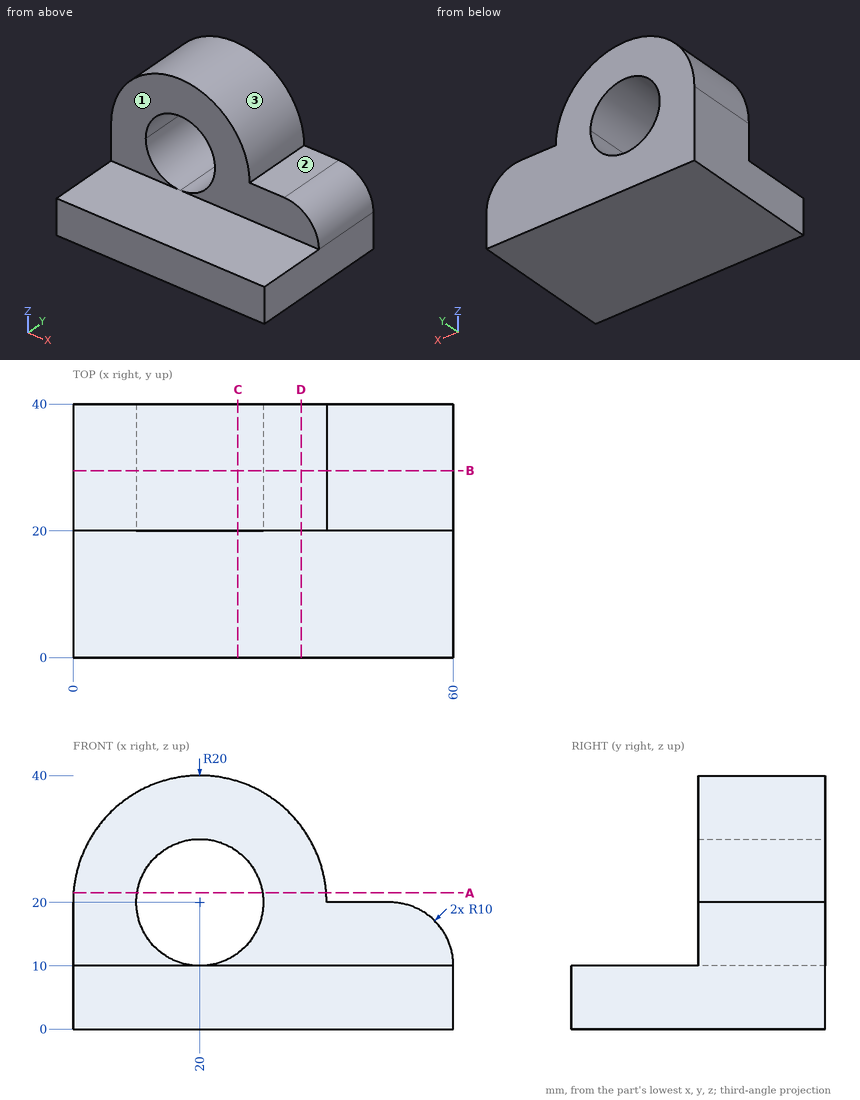
Geometry check sheet. Reference: drawing and pictorial views, mm from the part's lowest x, y, z. A direction names the side the tool comes from. Coordinates: 2 decimals unless noted, no trailing zeros. Order: outer loops, then holes, each group sorted by start corner. A loop starts at its lowest first (then second) coordinate and runs counter-clockwise, first axis right, second up.
Item 1: Section check A-A (z = 21.5). Enter the section's corners in (x, y), plus the area to 3 significant figures.
Item 2: Section check B-B (y = 29.5). Enter the section's corners in (x, z).
Item 3: Scan lines: line 1 along Y through (x, z) = (32, 26); line 2 along Z through (x, y) = (17, 22); line 3 along X through (y, z) = (21, 13). Record each from-to range of solid material in increasing order.
Item 4: Depth check by flat-ended pin: pin 1 (22 mm diameter, centred on x = 29.5, y = 13.5, fed in from +Z); pin 2 (1.5 mm diameter, centred on x = 49, y = 12.5, fed in from +Z); pin 3 (10 mm diameter, centred on y = 31, z = 16.5, fed in from +X); pin 4 (24 mm diameter, centred on x = 39.5, z = 18, fed in from -Y). Enter the tip coordinate at first touch or a pass-through.
Item 5: Tool access check on the marked faces 1, 2 and 3. Record the directions out of +Z, -Z, +X, -X, +Y, -Y that give a thin tool (end or side, any length) a straight path to the whole face; none if there is none.
Item 6: Section check D-D (x = 36). Enter the section's corners in (y, z).
Item 7: Section check C-C (x = 26). Enter the section's corners in (y, z).
Check sheet entries:
1. outline: (0.06, 20) - (10.11, 20) - (10.11, 40) - (0.06, 40) - close; (29.89, 20) - (39.94, 20) - (39.94, 40) - (29.89, 40) - close
1. area: 402 mm2
2. outline: (0, 0) - (60, 0) - (60, 10) arc R10 ccw to (50, 20) - (40, 20) arc R20 ccw to (0, 20) - close; hole circle Ø20 at (20, 20)
3. line 1: y = 20 to 40
3. line 2: z = 0 to 10.46, 29.54 to 39.77
3. line 3: x = 0 to 12.86, 27.14 to 59.54
4. pin 1: stops at z = 39.99
4. pin 2: stops at z = 10
4. pin 3: stops at x = 59.89
4. pin 4: stops at y = 0
5. face 1: +Z, +X, -X, -Y
5. face 2: +Z, +X, +Y, -Y
5. face 3: +Z, +Y, -Y
6. outline: (0, 0) - (40, 0) - (40, 32) - (20, 32) - (20, 10) - (0, 10) - close
7. outline: (0, 0) - (40, 0) - (40, 12) - (20, 12) - (20, 10) - (0, 10) - close; (20, 28) - (40, 28) - (40, 39.08) - (20, 39.08) - close
